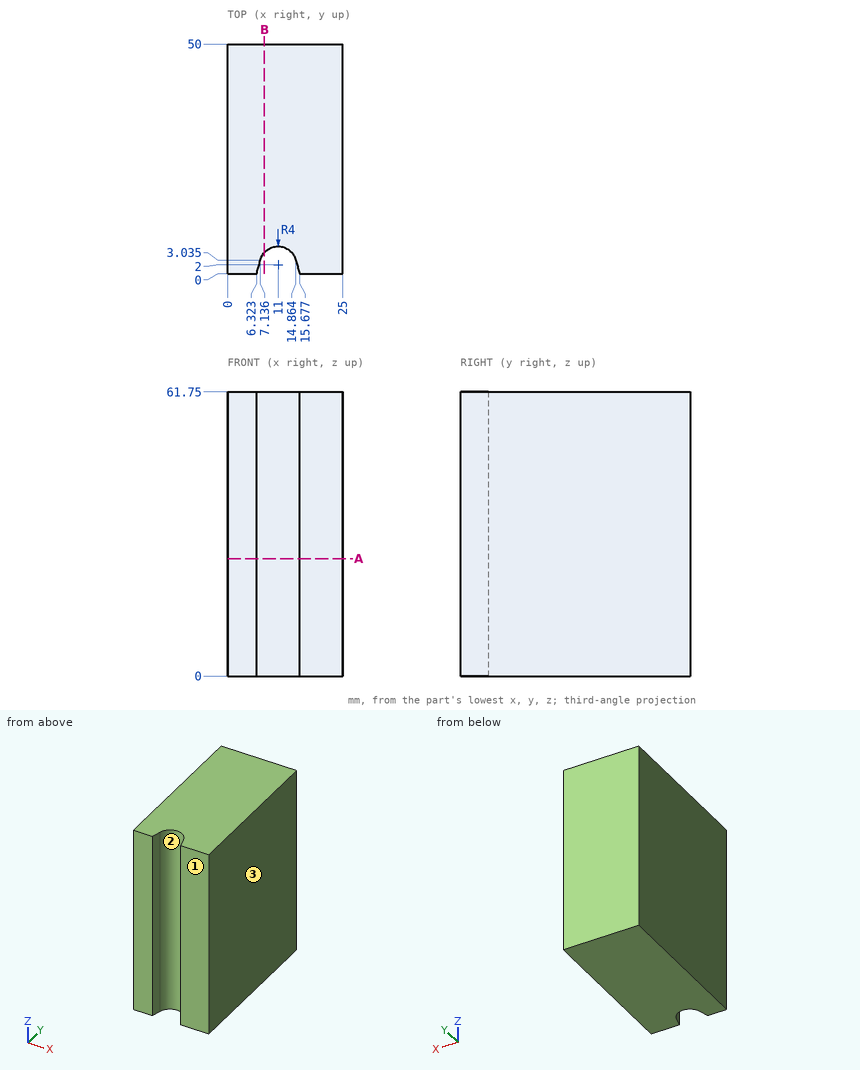
Can you work these out from the drawing? Everything is in mm from the part's minimum corner. Give positions to 0.01 mm unless a question says otherwise; leave off trailing zeros. Loops run counter-clockwise (first coordinate to the right, second up) from the corner with the lowest first, then second, coordinate; pieces in that order, holes last. Notation, with made-up numbers: (45, 37) - (95, 37) arc R15 ccw to (95, 51) - close; hole circle Ø2 at (26.25, 63.5). An arc over 180 degrees is marked (long way). Answer as a JSON object with one key per item and string values.
Q1. If we mould it in two halves opening along X, with no side actions, what happens to the marked faces 1, 2 and 3? For each: pulls with the +X half, pulls with the -X half, needs draft (parallel to the pull), parting line crosses it, or undercut.
Geometry says:
{"face 1": "needs draft", "face 2": "undercut", "face 3": "pulls with the +X half"}
Q2. Will this pin go through, and if not, where does the flat tip stop? P1, Ø10, axis at y = 26.5, z = 47, coming from the -X side.
Geometry says:
{"P1": "x = 0"}
Q3. Imagine slicing it at B-B on x = 8. Write out the boundary of the cut face in (y, z).
Geometry says:
{"outline": "(4.65, 0) - (50, 0) - (50, 61.75) - (4.65, 61.75) - close"}
Q4. Imagine slicing it at A-A on z = 25.5. Write out the boundary of the cut face in (x, y) (1 decimal), plus the area to 3 significant figures.
Geometry says:
{"outline": "(0, 0) - (6.3, 0) - (7.1, 3) arc R4 cw to (14.9, 3) - (15.7, 0) - (25, 0) - (25, 50) - (0, 50) - close", "area": "1,210 mm²"}
Q5. If I drill on L1, parallel to Y at x = 11, z = 33.5; L2, parallel to Y at x = 12.25, z = 36, over which ranges is the centre line in solid material (lowest first)?
Geometry says:
{"L1": "6 to 50", "L2": "5.8 to 50"}
